CAD build for the part. Positions are in the model's coordinates, mm. A direction names the side the tool comes from. Coordinates: 2 decimals unless noted, no trailing zeros. Write each loop counter-clockwise with the first axis right and the second up, starting at its lowest first coordinate (ties: lowest second). Pieces come first, ordered by that corner, then holes. Notation, with made-up numbers: (62, 28.5) - (112, 28.5) arc R37 ccw to (112, 64.5) - close; hole circle Ø11 at (19.5, 12). An arc over 180 degrees is marked (long way). Answer in a Markdown table with one row per item. Add a question column.
Q1. Two-plate mould, pull along X, no slides. Class faces 1 (the flat face through (23, -16, 0)), 2 (the flat face through (0, -6.35, -16)), 3 (the flat face through (31.75, -3, -3)), 4 (the flat face through (19.68, -24.76, -15.05)): +X half, -X half, draft (parallel to the pull), parting line (faces both ways), or undercut.
Q2. Band-saw the part on A-A (y = -20.75). List the corners of the cut face in (x, z), and give its area (3 significant figures).
Q3. 3-axis set-ups, long thin cutter, end or side, ignore diameter. For faces 5 (the flat face through (25.4, -16, -10)), 6 (the flat face through (15.467, -16, 12)), 7 (the flat face through (19.05, -15, -16)): which of +Z, -Z, +X, -X, +Y, -Y reach the whole face in a straight line?
Q4. Band-saw the part on B-B (z = -6.5). List the corners of the cut face in (x, y), and give its area (3 significant figures).
Q5. Band-saw the part on D-D (z = 16.5). List the corners of the cut face in (x, y).
Q6. Drill centre lines: line 1 along X through (y, z) = (-16, -15); line 2 along Z through (x, y) = (-24.5, -22.5); line 3 along Y through (x, z) = (29, 3). Where is each one in solid material? Low to high. Write a range as from..to.
Q7. Band-saw the part on C-C (x = 0). List the corners of the cut face in (y, z).
Q8. Pin check, flat tips, straight feed: pin 1 (5.5 mm diameter, centred on y = -12, z = -5.5, fed in from -X); pin 2 (12 mm diameter, centred on y = -19, z = 12.5, fed in from +X); pin 3 (2.5 mm diameter, centred on x = -22, y = -16, fed in from +Z). Stop position of each tip, or through.
```python
from build123d import *

# Parameters (mm, degrees)
F1_DEPTH = 6.35
F3_DEPTH = 19.05
F4_R     = 5.08
F5_SIZE  = 1.27


with BuildPart() as f1:
    # F0 (on Front) → F1 (new body)
    with BuildSketch(Plane.XZ):
        with BuildLine():
            Line((-12.7, 19.05), (-25.4, 19.05))
            ThreePointArc((-25.4, 19.05), (-29.890128, 17.190128), (-31.75, 12.7))
            Line((-31.75, 12.7), (-31.75, -19.05))
            Line((-31.75, -19.05), (31.75, -19.05))
            Line((31.75, -19.05), (31.75, 12.7))
            ThreePointArc((31.75, 12.7), (29.890128, 17.190128), (25.4, 19.05))
            Line((25.4, 19.05), (12.7, 19.05))
            ThreePointArc((12.7, 19.05), (0, 6.35), (-12.7, 19.05))
        make_face()
    extrude(amount=F1_DEPTH)

    # F2 (on face) → F3 (join)
    with BuildSketch(Plane.XZ.offset(6.35)):
        with BuildLine():
            ThreePointArc((12.7, 19.05), (0, 6.35), (-12.7, 19.05))
            Line((-12.7, 19.05), (-15.467166, 19.05))
            Line((-15.467166, 19.05), (-15.467166, 0))
            Line((-15.467166, 0), (-25.4, 0))
            Line((-25.4, 0), (-25.4, -19.05))
            Line((-25.4, -19.05), (-19.05, -19.05))
            Line((-19.05, -19.05), (-19.05, -12.423539))
            Line((-19.05, -12.423539), (19.05, -12.423539))
            Line((19.05, -12.423539), (19.05, -19.05))
            Line((19.05, -19.05), (25.4, -19.05))
            Line((25.4, -19.05), (25.4, 0))
            Line((25.4, 0), (15.467166, 0))
            Line((15.467166, 0), (15.467166, 19.05))
            Line((15.467166, 19.05), (12.7, 19.05))
        make_face()
    extrude(amount=F3_DEPTH)

    # F4
    f4_edges = [f1.edges().sort_by_distance(p)[0] for p in [
        (-15.467166, -15.875, 0),
        (15.467166, -15.875, 0),
    ]]
    fillet(f4_edges, radius=F4_R)

    # F5
    f5_edges = [f1.edges().sort_by_distance(p)[0] for p in [
        (0, -25.4, -12.423539),
        (-19.05, -25.4, -15.736769),
        (19.05, -25.4, -15.736769),
    ]]
    chamfer(f5_edges, length=F5_SIZE)


solid = f1.part
```
Checked values:
| question | item | result |
|---|---|---|
| 1 | face 1 | draft |
| 1 | face 2 | undercut |
| 1 | face 3 | +X half |
| 1 | face 4 | undercut |
| 2 | outline | (-25.4, -19.05) - (-19.05, -19.05) - (-19.05, -12.42) - (19.05, -12.42) - (19.05, -19.05) - (25.4, -19.05) - (25.4, 0) - (20.55, 0) arc R5.08 cw to (15.47, 5.08) - (15.47, 19.05) - (12.7, 19.05) arc R12.7 cw to (-12.7, 19.05) - (-15.47, 19.05) - (-15.47, 5.08) arc R5.08 cw to (-20.55, 0) - (-25.4, 0) - close |
| 2 | area | 1,060 mm² |
| 3 | face 5 | +Z, -Z, +X, -Y |
| 3 | face 6 | +Z, +X, -Y |
| 3 | face 7 | -Z, -Y |
| 4 | outline | (-31.75, -6.35) - (-25.4, -6.35) - (-25.4, -25.4) - (25.4, -25.4) - (25.4, -6.35) - (31.75, -6.35) - (31.75, 0) - (-31.75, 0) - close |
| 4 | area | 1,370 mm² |
| 5 | outline | (-30.49, -6.35) - (-15.47, -6.35) - (-15.47, -25.4) - (-12.44, -25.4) - (-12.44, 0) - (-30.49, 0) - close; (12.44, -25.4) - (15.47, -25.4) - (15.47, -6.35) - (30.49, -6.35) - (30.49, 0) - (12.44, 0) - close |
| 6 | line 1 | x = -25.4..-19.05, 19.05..25.4 |
| 6 | line 2 | z = -19.05..0 |
| 6 | line 3 | y = -6.35..0 |
| 7 | outline | (-25.4, -11.15) - (-24.13, -12.42) - (-6.35, -12.42) - (-6.35, -19.05) - (0, -19.05) - (0, 6.35) - (-25.4, 6.35) - close |
| 8 | pin 1 | stops at x = -25.4 |
| 8 | pin 2 | stops at x = 15.47 |
| 8 | pin 3 | stops at z = 0 |
